from build123d import *

# Parameters (mm, degrees)
F1_DEPTH = 6.35


with BuildPart() as f1:
    # F0 (on Top) → F1 (new body)
    with BuildSketch(Plane.XY):
        Polygon((101.6, 0), (6.35, 0), (6.35, -736.6), (50.8, -736.6), (101.6, -127), align=None)
        with BuildLine():
            ThreePointArc((19.05, -133.35), (22.225, -130.175), (25.4, -133.35))
            Line((25.4, -133.35), (25.4, -165.1))
            ThreePointArc((25.4, -165.1), (22.225, -168.275), (19.05, -165.1))
            Line((19.05, -165.1), (19.05, -133.35))
        make_face(mode=Mode.SUBTRACT)
    extrude(amount=F1_DEPTH)


with BuildPart() as f2_1:
    # F2: instance of F1
    add(f1.part.mirror(Plane.YZ))


solid = f2_1.part
Source: CAD feature listing. Evaluate the final solid. Frame: model axes, mm. Round coordinates to 2 decimals unless told otherwise and drop trailing zeros. Loops run counter-clockwise (first coordinate to the right, second up) from the corner with the lowest first, then second, coordinate; pieces in that order, holes last.
Q1. Ray query, line 1 (Y direction, x = -19.5, z = 1); line 2 (X direction, y = -482, z = 2); line 3 (X direction, y = -251.5, z = 1.75) (3 decimals). Return the intervals inside material, ascending.
Q2. Section A-A, the plane z = 4. Return loops of the section in (x, y) (3 decimals), plus the area to 3 significant figures.
Q3. First-contact query: P1, Ø2, axis at y = -300, z = 1, coming from the -X side; P2, Ø10, axis at x = -45, y = -582, coming from the -Z side; P3, Ø1.9, axis at y = -142.5, z = 4.5, coming from the -X side. Flat tips, straight axial feed; report the tip coordinate or a pass-through.
Q4. Section B-B, the plane y = -256. Return loops of the section in (x, z), plus the area to 3 significant figures.
Q5. Section C-C, the plane x = -64. Return loops of the section in (y, z), plus the area to 3 significant figures.
Solutions:
1. line 1: y = -736.6 to -166.73, -131.72 to 0
1. line 2: x = -72.02 to -6.35
1. line 3: x = -91.225 to -6.35
2. outline: (-101.6, -127) - (-50.8, -736.6) - (-6.35, -736.6) - (-6.35, 0) - (-101.6, 0) - close; hole (-25.4, -165.1) arc R3.175 ccw to (-19.05, -165.1) - (-19.05, -133.35) arc R3.175 ccw to (-25.4, -133.35) - close
2. area: 54,400 mm2
3. P1: stops at x = -87.27
3. P2: stops at z = 0
3. P3: stops at x = -100.39
4. outline: (-90.85, 0) - (-6.35, 0) - (-6.35, 6.35) - (-90.85, 6.35) - close
4. area: 537 mm2
5. outline: (-578.2, 0) - (0, 0) - (0, 6.35) - (-578.2, 6.35) - close
5. area: 3,670 mm2
